Read the model definition and answer for the solid it produces. Units are mm, in the model's axes. A direction names the side the tool comes from. Give positions to 0.01 mm unless a question says otherwise; leave off trailing zeros. Order: outer loops, then holes, each group sorted by start corner. A loop starts at its lowest first (then second) coordinate and runs counter-clockwise, first axis right, second up. Notation, with made-up numbers: (20, -2.5) -> (36, -2.5) arc R24 ccw to (36, 19.5) -> close; hole circle Ø4 at (80.5, 12). An arc over 180 degrees is marked (long way). One line per item, written item: value. Start each with the question number.
from build123d import *

# Parameters (mm, degrees)
F0_W     = 57.277
F0_H     = 72.7456
F0_W_2   = 44.577
F0_H_2   = 60.0456
F1_DEPTH = 20.32
F2_R     = 3.175
F3_R     = 2.54


with BuildPart() as f1:
    # F0 (on Front) → F1 (new body)
    with BuildSketch(Plane.XZ):
        Rectangle(F0_W, F0_H)
        Rectangle(F0_W_2, F0_H_2, mode=Mode.SUBTRACT)
    extrude(amount=F1_DEPTH)

    # F2
    f2_edges = [f1.edges().sort_by_distance(p)[0] for p in [
        (28.6385, -10.16, 36.3728),
        (28.6385, -10.16, -36.3728),
        (-28.6385, -10.16, -36.3728),
        (-28.6385, -10.16, 36.3728),
    ]]
    fillet(f2_edges, radius=F2_R)

    # F3
    f3_edges = [f1.edges().sort_by_distance(p)[0] for p in [
        (0, -20.32, 36.3728),
    ]]
    fillet(f3_edges, radius=F3_R)


solid = f1.part
Item 1: Find section A-A on x = -7. Write down the section's boundary in (y, z), then the cut area to 3 significant figures.
Item 2: A tool of negligible diameter and unlimited length cuts with its end or side. For faces 1 (the cylindrical face through (-0.356, -19.596, -35.609)), 2 (the flat face through (22.288, -10, 0)), from which of +Z, -Z, +X, -X, +Y, -Y can it reach the whole face along a straight path? Write none if from no direction.
Item 3: A flat-ended cylindrical pin translates along its axis: pin 1 (5 mm diameter, centred on x = -18, z = 5, fed in from +Y). Find the tip coordinate at first contact, or state that the pin passes through.
Item 4: Find section B-B on z = 22.5. Write down the section's boundary in (x, y).
Item 5: For a pull along Z with two mould halves and no side action, classify faces 3 (the cylindrical face through (0.356, -19.596, 35.609)), 4 (the flat face through (0, -9, -36.373)), 5 (the flat face through (0, -10, -30.023)) as +Z half, -Z half, draft (parallel to the pull), parting line (faces both ways), or undercut.
Item 6: Find the intervals of material crossed by line 1 (Z direction, x = -13, y = -16); line 2 (X direction, y = -7.5, z = 1.5); line 3 (Z direction, x = 5, y = -18.5), in increasing order. Write a range as from..to.
Checks:
1. outline: (-20.32, -33.83) arc R2.54 ccw to (-17.78, -36.37) -> (0, -36.37) -> (0, -30.02) -> (-20.32, -30.02) -> close; (-20.32, 30.02) -> (0, 30.02) -> (0, 36.37) -> (-17.78, 36.37) arc R2.54 ccw to (-20.32, 33.83) -> close
1. area: 255 mm2
2. face 1: -Z, +X, -X, -Y
2. face 2: +Y, -Y
3. pin 1: through
4. outline: (-28.64, -17.78) arc R2.54 ccw to (-26.1, -20.32) -> (-22.29, -20.32) -> (-22.29, 0) -> (-28.64, 0) -> close; (22.29, -20.32) -> (26.1, -20.32) arc R2.54 ccw to (28.64, -17.78) -> (28.64, 0) -> (22.29, 0) -> close
5. face 3: +Z half
5. face 4: -Z half
5. face 5: undercut
6. line 1: -36.37..-30.02, 30.02..36.37
6. line 2: -28.64..-22.29, 22.29..28.64
6. line 3: -36.27..-30.02, 30.02..36.27
